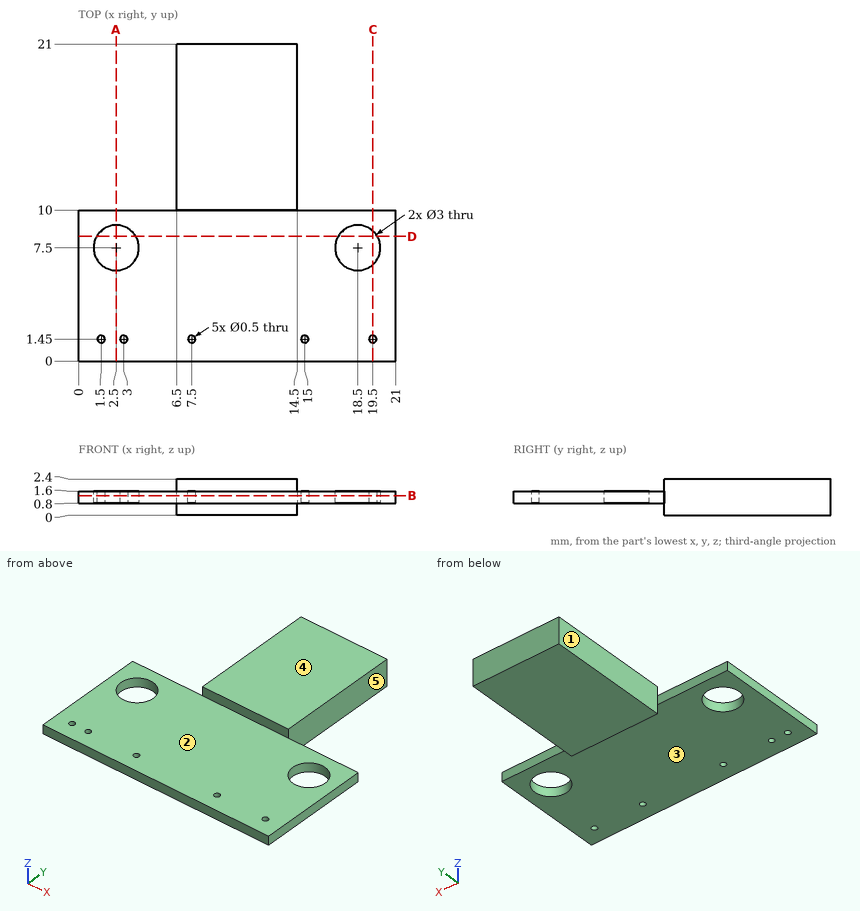
Input: dimensioned drawing with shaded views. Units: mm. Origin: part minimum x, y, z. A direction names the side the tool comes from. Round coordinates to 2 decimals unless told otherwise and drop trailing zeros. Order: outer loops, then holes, each group sorted by start corner. A loop starts at its lowest first (then second) coordinate and runs counter-clockwise, first axis right, second up. Notation, with made-up numbers: (-27.75, 25) - (3.25, 25) arc R21 cw to (3.25, 48) - close; hole circle Ø2 at (69, -6.5). An arc over 180 degrees is marked (long way). Use CSV: the item, a comma, the result in double quotes. Start each with the question number.
Q1. Section query D-D (y = 8.25). Return loops of the section in (x, z).
Q2. Section query C-C (x = 19.5). Return loops of the section in (y, z), and give its area (3 significant figures).
Q3. First-contact query: pin 1 (0.6 mm diameter, centred on x = 8.5, z = 2, fed in from -Y); pin 2 (0.6 mm diameter, centred on x = 3.5, z = 1, fed in from +Y); pin 3 (5 mm diameter, centred on x = 3, y = 9, fed in from +Z); pin 4 (8 mm diameter, centred on x = 4, y = 15, fed in from +Z). Flat tips, straight axial feed; report the tip coordinate or a pass-through.
Q4. Section query B-B (z = 1.3). Return loops of the section in (x, y), and give its area (3 significant figures).
Q5. Material intervals for line 1 along Y through (x, z) = (15, 1.3); line 2 along Y through (x, z) = (3, 1.15); line 3 along X through (y, z) = (1.25, 1.35), sorted ascending. Write a range as from..to.
Q6. Section query A-A (x = 2.5). Return loops of the section in (y, z).
Q7. Access query for the marked faces 1, 2, 3, 4 and 5. Directions: +Z, -Z, +X, -X, +Y, -Y. A direction counts if a zero-diameter tool reaches every point of the face in a straight line with its end or side. Return the directions, or none.
Result set:
1,outline,"(0, 0.8) - (1.2, 0.8) - (1.2, 1.6) - (0, 1.6) - close; (3.8, 0.8) - (17.2, 0.8) - (17.2, 1.6) - (3.8, 1.6) - close; (19.8, 0.8) - (21, 0.8) - (21, 1.6) - (19.8, 1.6) - close"
2,outline,"(0, 0.8) - (1.2, 0.8) - (1.2, 1.6) - (0, 1.6) - close; (1.7, 0.8) - (6.38, 0.8) - (6.38, 1.6) - (1.7, 1.6) - close; (8.62, 0.8) - (10, 0.8) - (10, 1.6) - (8.62, 1.6) - close"
2,area,"5.81 mm2"
3,pin 1,"stops at y = 10"
3,pin 2,"stops at y = 10"
3,pin 3,"stops at z = 1.6"
3,pin 4,"stops at z = 2.4"
4,outline,"(0, 0) - (21, 0) - (21, 10) - (14.5, 10) - (14.5, 21) - (6.5, 21) - (6.5, 10) - (0, 10) - close; hole circle Ø3 at (2.5, 7.5); hole circle Ø0.5 at (1.5, 1.45); hole circle Ø0.5 at (3, 1.45); hole circle Ø0.5 at (7.5, 1.45); hole circle Ø0.5 at (15, 1.45); hole circle Ø3 at (18.5, 7.5); hole circle Ø0.5 at (19.5, 1.45)"
4,area,"283 mm2"
5,line 1,"y = 0..1.2, 1.7..10"
5,line 2,"y = 0..1.2, 1.7..6.09, 8.91..10"
5,line 3,"x = 0..1.35, 1.65..2.85, 3.15..7.35, 7.65..14.85, 15.15..19.35, 19.65..21"
6,outline,"(0, 0.8) - (6, 0.8) - (6, 1.6) - (0, 1.6) - close; (9, 0.8) - (10, 0.8) - (10, 1.6) - (9, 1.6) - close"
7,face 1,"+Z, -Z, -X, +Y"
7,face 2,"+Z, +X, -X, -Y"
7,face 3,"-Z, +X, -X, -Y"
7,face 4,"+Z, +X, -X, +Y, -Y"
7,face 5,"+Z, -Z, +X, +Y"
